from build123d import *

# Parameters (mm, degrees)
SKETCH1_W           = 431.8
SKETCH1_H           = 95
SKETCH1_R           = 1.770184209
SKETCH1_R_2         = 1.902933344
SKETCH1_R_3         = 2
BOSS_EXTRUDE1_DEPTH = 3.175
FILLET1_R           = 10
SKETCH10_R          = 9.179936936
BOSS_EXTRUDE3_DEPTH = 3.175
SKETCH11_R          = 1.770587682
CUT_EXTRUDE5_DEPTH  = 3.175
CUT_EXTRUDE6_DEPTH  = 3.175
SKETCH13_R          = 11.741940518
BOSS_EXTRUDE4_DEPTH = 3.175
SKETCH14_R          = 1.762256498
CUT_EXTRUDE8_DEPTH  = 3.175


with BuildPart() as part:
    # Sketch1 → Boss-Extrude1 (new body)
    with BuildSketch(Plane(origin=(0, 0, 0), x_dir=(1, 0, 0), z_dir=(0, 1, 0))):
        with Locations((213.767466267, 47.5)):
            Rectangle(SKETCH1_W, SKETCH1_H)
        with Locations(Location((48.867466267, 40.050297191, 0), (0, 0, 270))):
            Circle(SKETCH1_R, mode=Mode.SUBTRACT)
        with Locations(Location((236.169368623, 16.995054431, 0), (0, 0, 270))):
            Circle(SKETCH1_R_2, mode=Mode.SUBTRACT)
        with Locations(Location((373.343160921, 26.368316597, 0), (0, 0, 270))):
            Circle(SKETCH1_R_3, mode=Mode.SUBTRACT)
    extrude(amount=BOSS_EXTRUDE1_DEPTH)

    # Fillet1
    fillet1_edges = [part.edges().sort_by_distance(p)[0] for p in [
        (-2.132533733, 1.5875, -95),
        (429.667466267, 1.5875, -95),
        (429.667466267, 1.5875, 0),
        (-2.132533733, 1.5875, 0),
    ]]
    fillet(fillet1_edges, radius=FILLET1_R)

    # Sketch10 → Boss-Extrude3 (add)
    with BuildSketch(Plane.XZ):
        with Locations((48.867466267, -40.050297191)):
            Circle(SKETCH10_R)
    extrude(amount=-BOSS_EXTRUDE3_DEPTH)

    # Sketch11 → Cut-Extrude5 (cut)
    with BuildSketch(Plane(origin=(0, 3.175, 0), x_dir=(1, 0, 0), z_dir=(0, 1, 0))):
        with Locations(Location((48.939345921, 40.088578466, 0), (0, 0, 270))):
            Circle(SKETCH11_R)
    extrude(amount=-CUT_EXTRUDE5_DEPTH, mode=Mode.SUBTRACT)

    # Sketch12 → Cut-Extrude6 (cut)
    with BuildSketch(Plane(origin=(0, 3.175, 0), x_dir=(1, 0, 0), z_dir=(0, 1, 0))):
        Polygon((48.341279917, 47.334727349), (48.341279917, 86.998039631), (12.939315235, 86.998039631), align=None)
        Polygon((44.60489186, 43.999769414), (9.202927178, 83.663081696), (6.684860974, 81.41555153), (6.684860974, 43.999769414), align=None)
        Polygon((44.60489186, 38.648134163), (6.684860974, 38.648134163), (6.684860974, 15.046824375), align=None)
        Polygon((7.853230038, 7.893935302), (48.341279917, 34.438493177), (48.341279917, 7.893935302), (44.60489186, 7.893935302), align=None)
        Polygon((55.459972177, 47.334727349), (90.838679195, 86.998039631), (55.459972177, 86.998039631), (53.759123425, 86.998039631), (53.759123425, 45.871199809), align=None)
        Polygon((90.838679195, 39.858977136), (90.838679195, 79.830290994), (55.833686687, 42.095331309), (55.833686687, 39.858977136), align=None)
        Polygon((53.759123425, 34.438493177), (53.759123425, 7.893935302), (90.838679195, 7.893935302), align=None)
        Polygon((61.64788979, 34.438493177), (90.838679195, 12.290395062), (90.838679195, 34.438493177), align=None)
    extrude(amount=-CUT_EXTRUDE6_DEPTH, mode=Mode.SUBTRACT)

    # Sketch13 → Boss-Extrude4 (add)
    with BuildSketch(Plane(origin=(0, 3.175, 0), x_dir=(1, 0, 0), z_dir=(0, 1, 0))):
        with Locations((48.939345921, 40.088578466)):
            Circle(SKETCH13_R)
    extrude(amount=-BOSS_EXTRUDE4_DEPTH)

    # Sketch14 → Cut-Extrude8 (cut)
    with BuildSketch(Plane(origin=(0, 3.175, 0), x_dir=(1, 0, 0), z_dir=(0, 1, 0))):
        with Locations(Location((48.870433526, 40.018247237, 0), (0, 0, 270))):
            Circle(SKETCH14_R)
    extrude(amount=-CUT_EXTRUDE8_DEPTH, mode=Mode.SUBTRACT)


solid = part.part
Check sheet for the modelled part. Datum: model origin and axes. Units: mm. A direction names the side the tool comes from. Round coordinates to 2 decimals unless told otherwise and drop trailing zeros. Loops run counter-clockwise (first coordinate to the right, second up) from the corner with the lowest first, then second, coordinate; pieces in that order, holes last. Notation, with made-up numbers: M 19.25,-22 L 67.25,-22 A9 ccw 67.25,-15 Z; hole C -27.5,-15.75 d3. An arc over 180 degrees is marked long. One line per item, written item: value.
(1) Sectioned sample at A-A, the plane z = -63. Record the cut outline in (x, y) (3 decimals).
Computed values:
outline: M -2.133,0 L 6.685,0 L 6.685,3.175 L -2.133,3.175 Z; M 27.646,0 L 34.359,0 L 34.359,3.175 L 27.646,3.175 Z; M 48.341,0 L 53.759,0 L 53.759,3.175 L 48.341,3.175 Z; M 69.433,0 L 75.226,0 L 75.226,3.175 L 69.433,3.175 Z; M 90.839,0 L 429.667,0 L 429.667,3.175 L 90.839,3.175 Z
(2) Access from +Z, -Z, +X, -X, +Y, -Y to the whole of each face (thin tool, end or side, straight path). Record for faces 1 (the face through (28.72, 1.61, -69.32)), 2 (the face through (0.719, 1.61, -91.993)).
Computed values:
face 1: +Y, -Y
face 2: -Z, -X, +Y, -Y
(3) Depth check by flat-ended pin: pin 1 Ø2.5 at (x, z) = (236.17, -17) entering from -Y; pin 2 Ø10 at (x, z) = (53, -22) entering from -Y. Enter the tip coordinate at first touch or a pass-through.
Computed values:
pin 1: passes through
pin 2: stops at y = 0
(4) Release check for a two-part mould opening along Z. For faces 3 (the face through (25.153, 1.61, -65.793)), 4 (the face through (0.719, 1.61, -3.007)), 5 (the face through (211, 3.175, -48)), 6 (the face through (75.253, 1.61, -63.029)) record: +Z half, -Z half, draft (parallel to the pull), parting line (faces both ways), or undercut.
Computed values:
face 3: undercut
face 4: +Z half
face 5: draft
face 6: undercut
(5) Thickness scan on line 1 (X direction, y = 2.95, z = -70); line 2 (X direction, y = 0.4, z = -69.5); line 3 (X direction, y = 0.35, z = -16). Record the ranges inside material, lowest first.
Computed values:
line 1: x = -2.13 to 6.68, 21.4 to 28.11, 48.34 to 53.76, 75.68 to 81.72, 90.84 to 429.67
line 2: x = -2.13 to 6.68, 21.84 to 28.56, 48.34 to 53.76, 75.23 to 81.26, 90.84 to 429.67
line 3: x = -2.13 to 6.68, 8.22 to 20.22, 48.34 to 53.76, 79.52 to 85.95, 90.84 to 234.55, 237.79 to 429.67
(6) Sectioned sample at B-B, the plane y = 2.05. Count the separate pieces of the cut face and the enclosed holes in it, then the cut area to 3 significant figures.
Computed values:
separate pieces: 1
enclosed holes: 11
area: 36,200 mm^2
